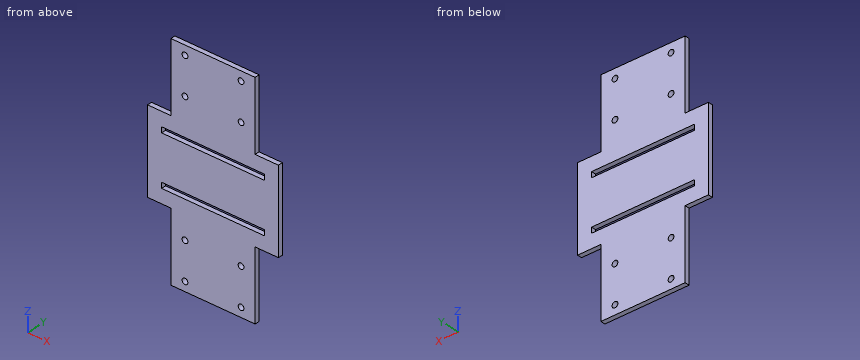
from build123d import *

# Parameters (mm, degrees)
EXTRUDE_1_DEPTH      = 5
SKETCH_3_W           = 30
SKETCH_3_H           = 90
CUT_EXTRUDE_2_DEPTH  = 5
SKETCH_5_W           = 30
SKETCH_5_H           = 90
CUT_EXTRUDE_3_DEPTH  = 5
SKETCH_7_W           = 90
SKETCH_7_H           = 20
EXTRUDE_2_DEPTH      = 5
SKETCH_9_W           = 90
SKETCH_9_H           = 20
EXTRUDE_3_DEPTH      = 5
SKETCH_10_R          = 3.1
CUT_EXTRUDE_4_DEPTH  = 5
SKETCH_11_R          = 3.1
CUT_EXTRUDE_5_DEPTH  = 5
SKETCH_12_R          = 3.1
CUT_EXTRUDE_7_DEPTH  = 5
SKETCH_13_R          = 3.1
CUT_EXTRUDE_8_DEPTH  = 5
SKETCH_14_W          = 100
SKETCH_14_H          = 6
CUT_EXTRUDE_9_DEPTH  = 5
SKETCH_15_W          = 100
SKETCH_15_H          = 6
CUT_EXTRUDE_10_DEPTH = 5
SKETCH_16_W          = 5
SKETCH_16_H          = 6
CUT_EXTRUDE_11_DEPTH = 5
SKETCH_17_W          = 5
SKETCH_17_H          = 6
CUT_EXTRUDE_12_DEPTH = 5
SKETCH_18_W          = 5
SKETCH_18_H          = 6
CUT_EXTRUDE_13_DEPTH = 5
SKETCH_19_W          = 5
SKETCH_19_H          = 6
CUT_EXTRUDE_14_DEPTH = 5


with BuildPart() as part:
    # 草图1 → 凸台-拉伸1 (new body)
    with BuildSketch(Plane(origin=(0, 0, 0), x_dir=(1, 0, 0), z_dir=(0, 1, 0))):
        Polygon((45, 45), (100, 45), (100, -45), (45, -45), (45, -100), (-45, -100), (-45, -45), (-100, -45), (-100, 45), (-45, 45), (-45, 100), (45, 100), align=None)
    extrude(amount=EXTRUDE_1_DEPTH)

    # 草图3 → 切除-拉伸2 (cut)
    with BuildSketch(Plane(origin=(0, 5, 0), x_dir=(1, 0, 0), z_dir=(0, 1, 0))):
        with Locations((-85, 0)):
            Rectangle(SKETCH_3_W, SKETCH_3_H)
    extrude(amount=-CUT_EXTRUDE_2_DEPTH, mode=Mode.SUBTRACT)

    # 草图5 → 切除-拉伸3 (cut)
    with BuildSketch(Plane(origin=(0, 5, 0), x_dir=(1, 0, 0), z_dir=(0, 1, 0))):
        with Locations((85, 0)):
            Rectangle(SKETCH_5_W, SKETCH_5_H)
    extrude(amount=-CUT_EXTRUDE_3_DEPTH, mode=Mode.SUBTRACT)

    # 草图7 → 凸台-拉伸2 (add)
    with BuildSketch(Plane(origin=(0, 5, 0), x_dir=(1, 0, 0), z_dir=(0, 1, 0))):
        with Locations((0, 110)):
            Rectangle(SKETCH_7_W, SKETCH_7_H)
    extrude(amount=-EXTRUDE_2_DEPTH)

    # 草图9 → 凸台-拉伸3 (add)
    with BuildSketch(Plane(origin=(0, 5, 0), x_dir=(1, 0, 0), z_dir=(0, 1, 0))):
        with Locations((0, -110)):
            Rectangle(SKETCH_9_W, SKETCH_9_H)
    extrude(amount=-EXTRUDE_3_DEPTH)

    # 草图10 → 切除-拉伸4 (cut)
    with BuildSketch(Plane(origin=(0, 5, 0), x_dir=(1, 0, 0), z_dir=(0, 1, 0))):
        with Locations(Location((-30, 110, 0), (0, 0, 270))):
            Circle(SKETCH_10_R)
        with Locations(Location((-30, 70, 0), (0, 0, 270))):
            Circle(SKETCH_10_R)
    extrude(amount=-CUT_EXTRUDE_4_DEPTH, mode=Mode.SUBTRACT)

    # 草图11 → 切除-拉伸5 (cut)
    with BuildSketch(Plane(origin=(0, 5, 0), x_dir=(1, 0, 0), z_dir=(0, 1, 0))):
        with Locations(Location((30, 110, 0), (0, 0, 270))):
            Circle(SKETCH_11_R)
        with Locations(Location((30, 70, 0), (0, 0, 270))):
            Circle(SKETCH_11_R)
    extrude(amount=-CUT_EXTRUDE_5_DEPTH, mode=Mode.SUBTRACT)

    # 草图12 → 切除-拉伸7 (cut)
    with BuildSketch(Plane(origin=(0, 5, 0), x_dir=(1, 0, 0), z_dir=(0, 1, 0))):
        with Locations(Location((-30, -110, 0), (0, 0, 270))):
            Circle(SKETCH_12_R)
        with Locations(Location((-30, -70, 0), (0, 0, 270))):
            Circle(SKETCH_12_R)
    extrude(amount=-CUT_EXTRUDE_7_DEPTH, mode=Mode.SUBTRACT)

    # 草图13 → 切除-拉伸8 (cut)
    with BuildSketch(Plane(origin=(0, 5, 0), x_dir=(1, 0, 0), z_dir=(0, 1, 0))):
        with Locations(Location((30, -110, 0), (0, 0, 270))):
            Circle(SKETCH_13_R)
        with Locations(Location((30, -70, 0), (0, 0, 270))):
            Circle(SKETCH_13_R)
    extrude(amount=-CUT_EXTRUDE_8_DEPTH, mode=Mode.SUBTRACT)

    # 草图14 → 切除-拉伸9 (cut)
    with BuildSketch(Plane(origin=(0, 5, 0), x_dir=(1, 0, 0), z_dir=(0, 1, 0))):
        with Locations((0, 27)):
            Rectangle(SKETCH_14_W, SKETCH_14_H)
    extrude(amount=-CUT_EXTRUDE_9_DEPTH, mode=Mode.SUBTRACT)

    # 草图15 → 切除-拉伸10 (cut)
    with BuildSketch(Plane(origin=(0, 5, 0), x_dir=(1, 0, 0), z_dir=(0, 1, 0))):
        with Locations((0, -27)):
            Rectangle(SKETCH_15_W, SKETCH_15_H)
    extrude(amount=-CUT_EXTRUDE_10_DEPTH, mode=Mode.SUBTRACT)

    # 草图16 → 切除-拉伸11 (cut)
    with BuildSketch(Plane(origin=(0, 5, 0), x_dir=(1, 0, 0), z_dir=(0, 1, 0))):
        with Locations((52.5, 27)):
            Rectangle(SKETCH_16_W, SKETCH_16_H)
    extrude(amount=-CUT_EXTRUDE_11_DEPTH, mode=Mode.SUBTRACT)

    # 草图17 → 切除-拉伸12 (cut)
    with BuildSketch(Plane(origin=(0, 5, 0), x_dir=(1, 0, 0), z_dir=(0, 1, 0))):
        with Locations((52.5, -27)):
            Rectangle(SKETCH_17_W, SKETCH_17_H)
    extrude(amount=-CUT_EXTRUDE_12_DEPTH, mode=Mode.SUBTRACT)

    # 草图18 → 切除-拉伸13 (cut)
    with BuildSketch(Plane(origin=(0, 5, 0), x_dir=(1, 0, 0), z_dir=(0, 1, 0))):
        with Locations((-52.5, 27)):
            Rectangle(SKETCH_18_W, SKETCH_18_H)
    extrude(amount=-CUT_EXTRUDE_13_DEPTH, mode=Mode.SUBTRACT)

    # 草图19 → 切除-拉伸14 (cut)
    with BuildSketch(Plane(origin=(0, 5, 0), x_dir=(1, 0, 0), z_dir=(0, 1, 0))):
        with Locations((-52.5, -27)):
            Rectangle(SKETCH_19_W, SKETCH_19_H)
    extrude(amount=-CUT_EXTRUDE_14_DEPTH, mode=Mode.SUBTRACT)


solid = part.part
Geometry check sheet. Reference: the model listing, model coordinates, mm. Round coordinates to 2 decimals unless told otherwise and drop trailing zeros. Write each loop counter-clockwise with the first axis right and the second up, starting at its lowest first coordinate (ties: lowest second). Pieces come first, ordered by that corner, then holes. Notation, with made-up numbers: (18, 3) - (50, 3) arc R35 cw to (50, 41) - close; hole circle Ø10 at (-16, 11.5). An arc over 180 degrees is marked (long way). One line per item, written item: value.
1. Cross-section at B-B on z = 70. Record the boundary of the cut face in (x, y).
The answers:
outline: (-45, 0) - (-33.1, 0) - (-33.1, 5) - (-45, 5) - close; (-26.9, 0) - (26.9, 0) - (26.9, 5) - (-26.9, 5) - close; (33.1, 0) - (45, 0) - (45, 5) - (33.1, 5) - close
2. Cross-section at C-C on y = 1.65. Give the number of separate pieces and of enclosed holes in the cut face, and give its area (3 significant figures).
The answers:
separate pieces: 1
enclosed holes: 10
area: 24,500 mm^2
3. Cross-section at A-A on x = 30. Record the boundary of the cut face in (y, z).
The answers:
outline: (0, -120) - (5, -120) - (5, -113.1) - (0, -113.1) - close; (0, -106.9) - (5, -106.9) - (5, -73.1) - (0, -73.1) - close; (0, -66.9) - (5, -66.9) - (5, -30) - (0, -30) - close; (0, -24) - (5, -24) - (5, 24) - (0, 24) - close; (0, 30) - (5, 30) - (5, 66.9) - (0, 66.9) - close; (0, 73.1) - (5, 73.1) - (5, 106.9) - (0, 106.9) - close; (0, 113.1) - (5, 113.1) - (5, 120) - (0, 120) - close
4. Scan lines: L1, parallel to Z at x = -0.5, y = 0.45; L2, parallel to X at y = 2.85, z = -70; L3, parallel to Z at x = 47, y = 4.2. Record each from-to range of solid material in increasing order.
The answers:
L1: z = -120 to -30, -24 to 24, 30 to 120
L2: x = -45 to -33.1, -26.9 to 26.9, 33.1 to 45
L3: z = -45 to -30, -24 to 24, 30 to 45
5. Cross-section at D-D on x = -15.5. Record the boundary of the cut face in (y, z).
The answers:
outline: (0, -120) - (5, -120) - (5, -30) - (0, -30) - close; (0, -24) - (5, -24) - (5, 24) - (0, 24) - close; (0, 30) - (5, 30) - (5, 120) - (0, 120) - close
6. Depth check by flat-ended pin: pin 1 Ø8 at (x, z) = (-30, 70) entering from +Y; pin 2 Ø1.5 at (y, z) = (2, 91) entering from +X; pin 3 Ø5 at (x, z) = (30, 70) entering from -Y; pin 4 Ø1.5 at (x, y) = (-49, 2.5) entering from -Z. Enter the tip coordinate at first touch or a pass-through.
The answers:
pin 1: stops at y = 5
pin 2: stops at x = 45
pin 3: passes through
pin 4: stops at z = -45
